Geometry: final body of the model. Coordinates: model frame, mm. Give positions to 0.01 mm unless a question says otherwise; leave off trailing zeros. Order: outer loops, then holes, each group sorted by start corner. A loop starts at its lowest first (then second) coordinate and runs counter-clockwise, first axis right, second up. Notation, with made-up numbers: M 78,78 L 137,78 A18 ccw 137,82 Z; hole C -31.75,60 d6. An arc over 180 degrees is marked long. Use CSV: the item, a comma, the result in double quotes.
```python
from build123d import *

# Parameters (mm, degrees)
PAD034_DEPTH  = 3
SKETCH060_R   = 2.9
HOLE001_DEPTH = 4.001


with BuildPart() as part:
    # Sketch058 → Pad034 (new body)
    with BuildSketch(Plane.XY.offset(-58.5)):
        Polygon((111, 40), (81, 40), (81, 1), (66.5, 1), (66.5, -43), (111, -43), align=None)
    extrude(amount=PAD034_DEPTH)

    # Sketch060 → Hole001 (cut, through all)
    with BuildSketch(Plane(origin=(1, 0, -54.5), x_dir=(1, 0, 0), z_dir=(0, 0, 1))):
        with Locations((95, 18)):
            Circle(SKETCH060_R)
        with Locations((82, -21)):
            Circle(SKETCH060_R)
        with Locations((95, -34)):
            Circle(SKETCH060_R)
    extrude(amount=-HOLE001_DEPTH, mode=Mode.SUBTRACT)


with BuildPart() as part_1:
    # Body014 placement: moved
    add(part.part.moved(Location((18.5, 0, 0))))


solid = part_1.part
```
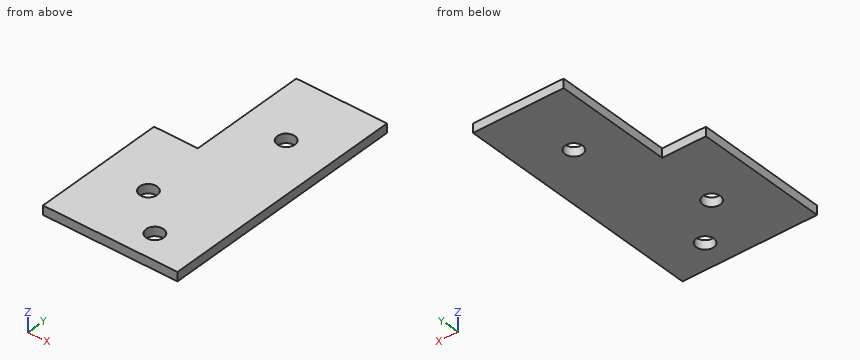
1. Line query: line 1 (Y direction, x = 114.5, z = -57.45); line 2 (Y direction, x = 101.5, z = -57.1); line 3 (Y direction, x = 88.5, z = -58.1). Output: solid intervals per line, ascending.
Answer:
line 1,"-43 to -36.9, -31.1 to 15.1, 20.9 to 40"
line 2,"-43 to -23.9, -18.1 to 40"
line 3,"-43 to 1"
2. Pin query (flat end, axial travel): pin 1 Ø1.5 at (x, z) = (92.5, -57) entering from +Y; pin 2 Ø0.9 at (y, z) = (23, -56.5) entering from -X; pin 3 Ø6.5 at (x, y) = (101.5, -21) entering from +Z. Return the tip coordinate at first contact, or that it passes through.
Answer:
pin 1,"y = 1"
pin 2,"x = 99.5"
pin 3,"z = -55.5"
3. Section A-A, the plane y = -34. Return the cut outline in (x, z).
Answer:
outline,"M 85,-58.5 L 111.6,-58.5 L 111.6,-55.5 L 85,-55.5 Z; M 117.4,-58.5 L 129.5,-58.5 L 129.5,-55.5 L 117.4,-55.5 Z"
4. Section B-B, the plane x = 114.5. Return the cut outline in (y, z), plus the area to 3 significant figures.
Answer:
outline,"M -43,-58.5 L -36.9,-58.5 L -36.9,-55.5 L -43,-55.5 Z; M -31.1,-58.5 L 15.1,-58.5 L 15.1,-55.5 L -31.1,-55.5 Z; M 20.9,-58.5 L 40,-58.5 L 40,-55.5 L 20.9,-55.5 Z"
area,"214 mm2"
5. Section D-D, the plane y = 18. Return the cut outline in (x, z), plus the area to 3 significant figures.
Answer:
outline,"M 99.5,-58.5 L 111.6,-58.5 L 111.6,-55.5 L 99.5,-55.5 Z; M 117.4,-58.5 L 129.5,-58.5 L 129.5,-55.5 L 117.4,-55.5 Z"
area,"72.6 mm2"
6. Section C-C, the plane z = -56.75. Return the cut outline in (x, y), plus the area to 3 significant figures.
Answer:
outline,"M 85,-43 L 129.5,-43 L 129.5,40 L 99.5,40 L 99.5,1 L 85,1 Z; hole C 101.5,-21 d5.8; hole C 114.5,-34 d5.8; hole C 114.5,18 d5.8"
area,"3,050 mm2"
